The listing builds one solid part. Answer for the finished solid, in the listing's coordinates (mm). Face numbers are marked on the shaded views. A direction names the side the tool comes from. Coordinates: 2 decimals unless noted, no trailing zeros. Loops run counter-clockwise (first coordinate to the right, second up) from the corner with the lowest first, then second, coordinate; pieces in that order, holes last. Notation, with made-up numbers: M -23,45 L 21,45 A26 ccw 21,64 Z; hole C -0.75,8.25 d2. An arc over 180 degrees is marked long. Answer as a JSON object with one key per item and string values. Group by question number.
1. Straight lines are drawn through the part: L1, parallel to X at y = 8, z = -4.5; L2, parallel to Z at x = 3, y = 9.5; L3, parallel to X at y = -21, z = 8.75. For each, find the intervals that lie inside material, in ascending order.
2. Determine the mould class of the marked faces 4, 5 and 6 for opening direction Y: released by +Y, released by -Y, zero draft, split by the parting line, or undercut.
3. A cutting plane is placed at B-B on z = 0. State how many separate pieces and enclosed holes the cut face has, and give its area (3 significant figures).
4. For the marked faces 1, 2 and 3, determine the directions among +Z, -Z, +X, -X, +Y, -Y from which every point of the face is accessible in a straight line to the end or side of a thin tool.
5. Given pin 1 (2.5 mm diameter, centred on x = 2.5, y = 9, fed in from +Z); pin 2 (2.5 mm diameter, centred on x = 2, z = 7.5, fed in from +Y); pin 3 (2.5 mm diameter, centred on x = 2.5, y = 10, fed in from -Z); pin 4 (2 mm diameter, centred on y = 9.5, z = 0, fed in from -X), each flat-ended and moving along its own axis, determine where each tip first touches the part or whether it passes through.
6. A cutting plane is placed at A-A on x = 2.75. Give the vertices of the cut face in (y, z).
7. A cutting plane is placed at C-C on y = 9.5. Give the vertices of the cut face in (x, z), and give its area (3 significant figures).
8. A cutting plane is placed at D-D on x = -2.75. Give the vertices of the cut face in (y, z), and give its area (3 significant figures).
from build123d import *

# Parameters (mm, degrees)
EXTRUDE_1_DEPTH             = 10
EXTRUDE_2_REACH             = 34.619
SKETCH_2_R                  = 10
EXTRUDE_2_DIRECTION_2_DEPTH = 2
SKETCH_4_R                  = 2.95
EXTRUDE_3_DEPTH             = 5
SKETCH_5_R                  = 1.5
CUT_EXTRUDE_1_DEPTH         = 44.874821937
SKETCH_6_R                  = 1.65
SKETCH_6_W                  = 14.704506527
SKETCH_6_H                  = 8.520368268
CUT_EXTRUDE_2_DEPTH         = 43.983979574
FILLET_1_R                  = 1
FILLET_2_R                  = 0.5


with BuildPart() as part:
    # 草图1 → 凸台-拉伸1 (new, symmetric)
    with BuildSketch(Plane.XY):
        with BuildLine():
            Line((-1.15, 3.987480407), (-1.15, 12))
            Line((-1.15, 12), (-4.15, 12))
            Line((-4.15, 12), (-4.15, 4.333301282))
            ThreePointArc((-4.15, 4.333301282), (-4.784308974, 3.620826928), (-5.297685557, 2.816829377))
            Line((-5.297685557, 2.816829377), (-8, -2.265484914))
            Line((-8, -2.265484914), (-8, -30))
            Line((-8, -30), (0, -30))
            Line((0, -30), (0, -8.485281374))
            Line((0, -8.485281374), (4.242640687, -4.242640687))
            ThreePointArc((4.242640687, -4.242640687), (5.999649956, 0.064810571), (4.15, 4.333301282))
            Line((4.15, 4.333301282), (4.15, 12))
            Line((4.15, 12), (1.15, 12))
            Line((1.15, 12), (1.15, 3.987480407))
            ThreePointArc((1.15, 3.987480407), (0, -4.15), (-1.15, 3.987480407))
        make_face()
    extrude(amount=EXTRUDE_1_DEPTH, both=True)

    # 凸台-拉伸2: up to this face of the body (flat: up to its plane)
    extrude_2_end = Plane(part.part.faces().sort_by_distance((-8, -16.132742457, 0))[0])
    # 草图2 → 凸台-拉伸2 (add, up to the picked face)
    with BuildSketch(Plane(origin=(0, 0, 0), x_dir=(0, 0, -1), z_dir=(1, 0, 0)), mode=Mode.PRIVATE) as extrude_2_sk1:
        with Locations((0, -30)):
            Circle(SKETCH_2_R)
    extrude_2_tool1 = split(extrude(extrude_2_sk1.sketch, amount=-EXTRUDE_2_REACH, mode=Mode.PRIVATE), bisect_by=extrude_2_end, keep=Keep.BOTH, mode=Mode.PRIVATE)
    add(extrude_2_tool1.solids().sort_by(Axis((0, -30, 0), (-1, 0, 0)))[0])

    # 草图2 → 凸台-拉伸2 direction 2 (add)
    with BuildSketch(Plane(origin=(0, 0, 0), x_dir=(0, 0, -1), z_dir=(1, 0, 0))):
        with Locations((0, -30)):
            Circle(SKETCH_2_R)
    extrude(amount=EXTRUDE_2_DIRECTION_2_DEPTH)

    # 草图4 → 凸台-拉伸3 (add)
    with BuildSketch(Plane(origin=(2, 0, 0), x_dir=(0, 0, -1), z_dir=(1, 0, 0))):
        with Locations((0, -30)):
            Circle(SKETCH_4_R)
    extrude(amount=EXTRUDE_3_DEPTH)

    # 草图5 → 切除-拉伸1 (cut, through all)
    with BuildSketch(Plane(origin=(7, 0, 0), x_dir=(0, 0, -1), z_dir=(1, 0, 0))):
        with Locations((0, -30)):
            Circle(SKETCH_5_R)
    extrude(amount=-CUT_EXTRUDE_1_DEPTH, mode=Mode.SUBTRACT)

    # 草图6 → 切除-拉伸2 (cut, through all)
    with BuildSketch(Plane(origin=(4.15, 0, 0), x_dir=(0, 0, -1), z_dir=(1, 0, 0))):
        with Locations(Location((0, 9.5, 0), (0, 0, 90))):
            Circle(SKETCH_6_R)
        with Locations((-12.852253263, 11.760184134)):
            Rectangle(SKETCH_6_W, SKETCH_6_H)
        with Locations((12.852253263, 11.760184134)):
            Rectangle(SKETCH_6_W, SKETCH_6_H)
    extrude(amount=-CUT_EXTRUDE_2_DEPTH, mode=Mode.SUBTRACT)

    # 圆角1
    fillet_1_edges = [part.edges().sort_by_distance(p)[0] for p in [
        (2.65, 7.5, -10),
        (-2.65, 7.5, -10),
        (2.65, 7.5, 10),
        (-2.65, 7.5, 10),
        (2.65, 12, 5.5),
        (-2.65, 12, 5.5),
        (2.65, 12, -5.5),
        (-2.65, 12, -5.5),
    ]]
    fillet(fillet_1_edges, radius=FILLET_1_R)

    # 圆角2
    fillet_2_edges = [part.edges().sort_by_distance(p)[0] for p in [
        (-2.65, 7.5, 5.5),
        (2.65, 7.5, 5.5),
        (2.65, 7.5, -5.5),
        (-2.65, 7.5, -5.5),
    ]]
    fillet(fillet_2_edges, radius=FILLET_2_R)


solid = part.part
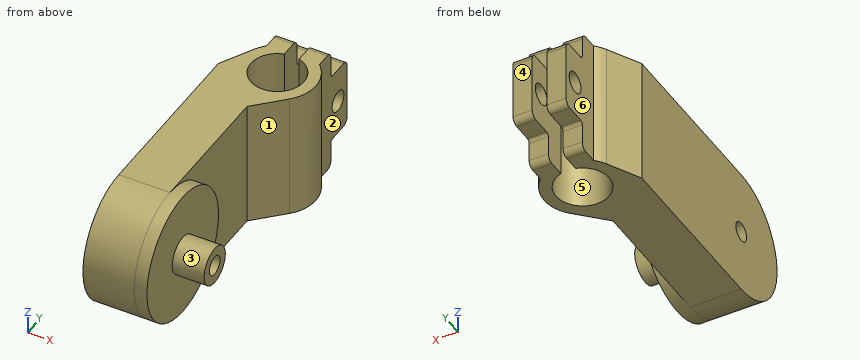
From the geometry:
{
 "1": {"L1": "x = -4.15 to -1.15, 1.15 to 4.15", "L2": "z = -5.5 to -1.65, 1.65 to 5.5", "L3": "x = -8 to 0"},
 "2": {"face 4": "released by +Y", "face 5": "undercut", "face 6": "zero draft"},
 "3": {"separate pieces": "4", "enclosed holes": "0", "area": "395 mm²"},
 "4": {"face 1": "+Z, -Z, +X", "face 2": "+Z, -Z, +X, +Y", "face 3": "+X"},
 "5": {"pin 1": "stops at z = 5.57", "pin 2": "stops at y = 7.5", "pin 3": "stops at z = -5.5", "pin 4": "passes through"},
 "6": {"outline": "C -30,0 d5.9; M -5.74,-10 L -3.11,-10 L -3.11,10 L -5.74,10 Z; M 3.11,-10 L 6.5,-10 A1 ccw 7.5,-9 L 7.5,-6 A0.5 cw 8,-5.5 L 11,-5.5 A1 ccw 12,-4.5 L 12,4.5 A1 ccw 11,5.5 L 8,5.5 A0.5 cw 7.5,6 L 7.5,9 A1 ccw 6.5,10 L 3.11,10 Z; hole C -30,0 d3; hole C 9.5,0 d3.3"},
 "7": {"outline": "M -4.15,-5.5 L -1.15,-5.5 L -1.15,-1.65 L -4.15,-1.65 Z; M -4.15,1.65 L -1.15,1.65 L -1.15,5.5 L -4.15,5.5 Z; M 1.15,-5.5 L 4.15,-5.5 L 4.15,-1.65 L 1.15,-1.65 Z; M 1.15,1.65 L 4.15,1.65 L 4.15,5.5 L 1.15,5.5 Z", "area": "46.2 mm²"},
 "8": {"outline": "M -30,-10 L -3.11,-10 L -3.11,10 L -30,10 A10 ccw Z; M 3.11,-10 L 6.5,-10 A1 ccw 7.5,-9 L 7.5,-6 A0.5 cw 8,-5.5 L 11,-5.5 A1 ccw 12,-4.5 L 12,4.5 A1 ccw 11,5.5 L 8,5.5 A0.5 cw 7.5,6 L 7.5,9 A1 ccw 6.5,10 L 3.11,10 Z; hole C -30,0 d3; hole C 9.5,0 d3.3", "area": "816 mm²"}
}
